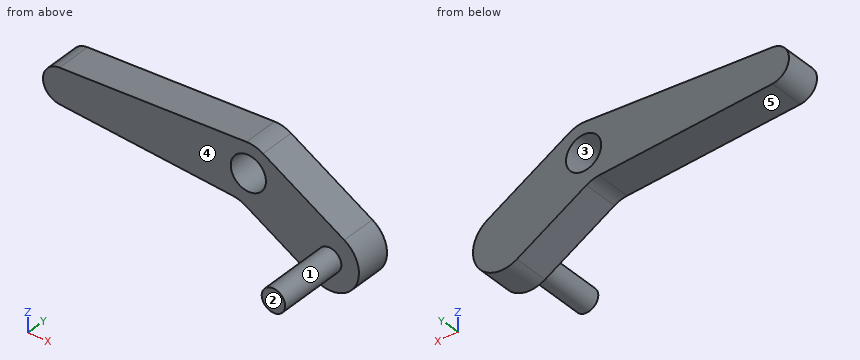
```python
from build123d import *

# Parameters (mm, degrees)
F0_R     = 1.5
F1_DEPTH = 3
F2_R     = 1
F3_DEPTH = 6


with BuildPart() as f1:
    # F0 (on Front) → F1 (new body)
    with BuildSketch(Plane.XZ):
        with BuildLine():
            Line((8.178203, -1.834936), (1.25, 2.165064))
            ThreePointArc((1.25, 2.165064), (0.571231, 2.433864), (-0.15625, 2.495112))
            Line((-0.15625, 2.495112), (-16.09375, 1.497067))
            ThreePointArc((-16.09375, 1.497067), (-17.5, 0), (-16.09375, -1.497067))
            Line((-16.09375, -1.497067), (-1.327463, -2.421768))
            ThreePointArc((-1.327463, -2.421768), (-0.761482, -2.523477), (-0.233713, -2.751817))
            Line((-0.233713, -2.751817), (5.678203, -6.165064))
            ThreePointArc((5.678203, -6.165064), (9.093267, -5.25), (8.178203, -1.834936))
        make_face()
        Circle(F0_R, mode=Mode.SUBTRACT)
    extrude(amount=F1_DEPTH)

    # F2 (on face) → F3 (join)
    with BuildSketch(Plane.XZ.offset(3)):
        with Locations((6.928203, -4)):
            Circle(F2_R)
    extrude(amount=F3_DEPTH)


solid = f1.part
```
Here's how the part is built. I have some questions about the finished solid (model axes, mm). Face numbers are marked on the shaded views. A direction names the side the tool comes from. Give positions to 0.01 mm unless a question says otherwise; leave off trailing zeros. Loops run counter-clockwise (first coordinate to the right, second up) from the corner with the lowest first, then second, coordinate; pieces in that order, holes last. Notation, with made-up numbers: M -36,89 L 21,89 A24 cw 21,114 Z; hole C 88,10 d7. An arc over 180 degrees is marked long. Use one line per item in the form item = value. Start each with the question number.
Q1. Thinking about a two-plate mould opening in X: for the marked faces 3, 4 and 5, which applies, +X half, -X half, draft (parallel to the pull), parting line (faces both ways), or undercut?
Q2. Which directions (+Z, -Z, +X, -X, +Y, -Y) give clear straight access to the entire face, cutting with the end or side of a thin tool? Please do the marked faces 1 and 2.
Q3. If we section it at A-A (z = -1): Write out the boundary of the cut face in (x, y), then the cut area to 3 significant figures.
Q4. I need wall thicknesses on line 1 along Y through (x, z) = (-16, 1); line 2 along Z through (x, y) = (0, -0.7); line 3 along Z through (x, y) = (-0.25, -1.5). Which ranges of each line are inside material? Lowest first, please.
Q5. If we section it at D-D (z = 1): Write out the boundary of the cut face in (x, y), then the cut area to 3 significant figures.
Q6. If we section it at C-C (z = -4): Write out the boundary of the cut face in (x, y), then the cut area to 3 significant figures.
Q7. Will these pins go through, and if not, where does the flat tip stop? pin 1 Ø1 at (x, y) = (-6, -1) entering from +Z; pin 2 Ø5 at (x, z) = (0, 0) entering from -Y.
Q8. If we section it at B-B (y = -4.75): Write out the boundary of the cut face in (x, z), then the cut area to 3 significant figures.
Taken from the geometry:
q1.face_3 = undercut
q1.face_4 = draft
q1.face_5 = -X half
q2.face_1 = -Y
q2.face_2 = +Z, -Z, +X, -X, -Y
q3.outline = M -17.12,-3 L -1.12,-3 L -1.12,0 L -17.12,0 Z; M 1.12,-3 L 6.73,-3 L 6.73,0 L 1.12,0 Z
q3.area = 64.8 mm^2
q4.line_1 = -3 to 0
q4.line_2 = -2.89 to -1.5, 1.5 to 2.5
q4.line_3 = -2.74 to -1.48, 1.48 to 2.49
q5.outline = M -17.12,-3 L -1.12,-3 L -1.12,0 L -17.12,0 Z; M 1.12,-3 L 3.27,-3 L 3.27,0 L 1.12,0 Z
q5.area = 54.4 mm^2
q6.outline = M 1.93,-3 L 5.93,-3 L 5.93,-9 L 7.93,-9 L 7.93,-3 L 9.43,-3 L 9.43,0 L 1.93,0 Z
q6.area = 34.5 mm^2
q7.pin_1 = 2.16
q7.pin_2 = -3
q8.outline = C 6.93,-4 d2
q8.area = 3.14 mm^2
